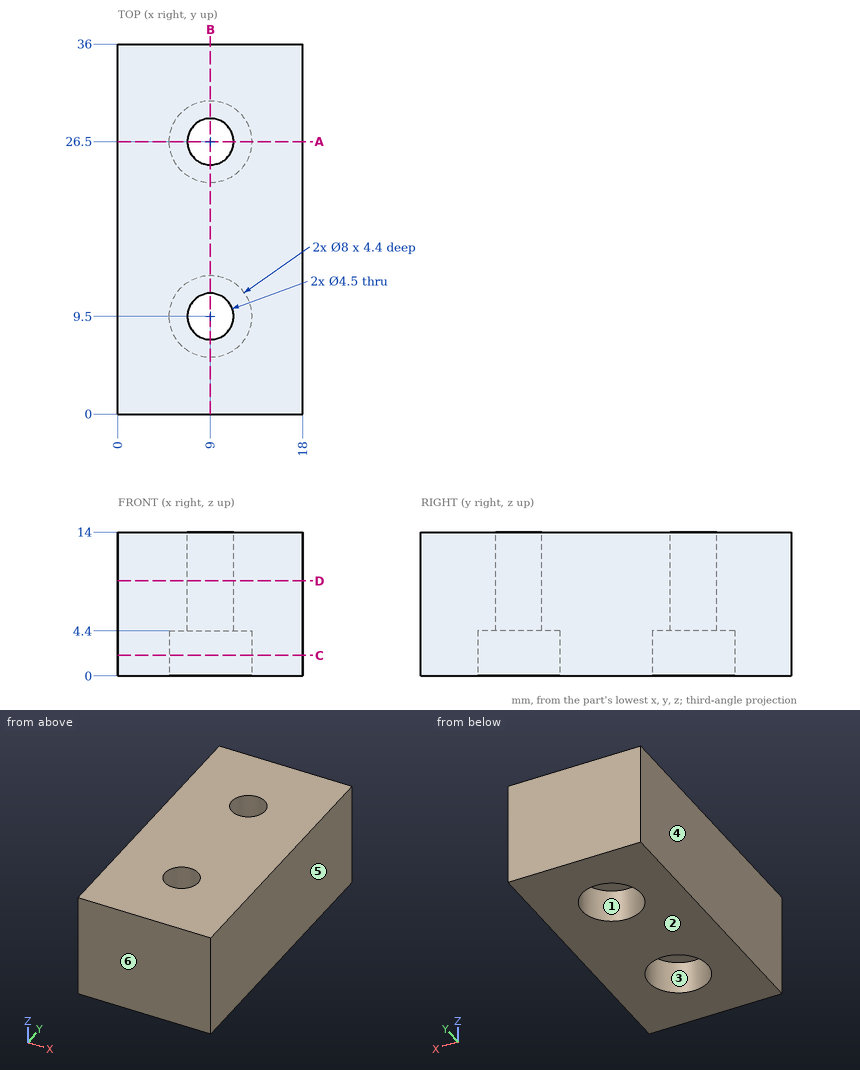
The figure shows three views and two pictorial views of one solid part (mm, origin at its lowest corner). Answer the questions. A direction names the side the tool comes from. Round coordinates to 2 decimals unless told otherwise and drop trailing zeros. Write each loop counter-clockwise with the first axis right and the second up, starting at its lowest first coordinate (ties: lowest second). Pieces come first, ordered by that corner, then holes. Notation, with made-up numbers: (-30, 0.5) -> (8, 0.5) arc R19 cw to (8, 25.5) -> close; hole circle Ø11 at (18.25, 37.5). An arc over 180 degrees is marked (long way). Answer as a JSON object with one key per item and string values. Group by question number.
Q1. Section A-A (y = 26.5) is taken. Write down the section's boundary in (x, z).
Q2. Which of the six approach directions +Z, -Z, +X, -X, +Y, -Y give full straight-line access (tool end or side, diameter ignored) to the marked faces 1 and 2?
Q3. This flat-tipped pin is pushed along its axis until it touches: pin 1 Ø7 at (x, y) = (9, 26.5) entering from -Z. Where does it stop, or does it pass through?
Q4. Section C-C (z = 2) is taken. Write down the section's boundary in (x, y).
Q5. Determine the mould class of the marked faces 3, 4, 5 and 6 for opening direction X: pulls with the +X half, pulls with the -X half, needs draft (parallel to the pull), parting line crosses it, or undercut.
Q6. Section B-B (x = 9) is taken. Write down the section's boundary in (y, z).
Q7. Section D-D (z = 9.25) is taken. Write down the section's boundary in (x, y), plus the area to 3 significant figures.
Q8. Straight lines are drawn through the part: line 1 along Y through (x, z) = (9, 2.05); line 2 along Y through (x, z) = (9, 9.5); line 3 along X through (y, z) = (29.5, 1.75). For each, find the intervals that lie inside material, in ascending order.
Check values:
{
 "1": {"outline": "(0, 0) -> (5, 0) -> (5, 4.4) -> (6.75, 4.4) -> (6.75, 14) -> (0, 14) -> close; (11.25, 4.4) -> (13, 4.4) -> (13, 0) -> (18, 0) -> (18, 14) -> (11.25, 14) -> close"},
 "2": {"face 1": "-Z", "face 2": "-Z, +X, -X, +Y, -Y"},
 "3": {"pin 1": "z = 4.4"},
 "4": {"outline": "(0, 0) -> (18, 0) -> (18, 36) -> (0, 36) -> close; hole circle Ø8 at (9, 9.5); hole circle Ø8 at (9, 26.5)"},
 "5": {"face 3": "undercut", "face 4": "pulls with the -X half", "face 5": "pulls with the +X half", "face 6": "needs draft"},
 "6": {"outline": "(0, 0) -> (5.5, 0) -> (5.5, 4.4) -> (7.25, 4.4) -> (7.25, 14) -> (0, 14) -> close; (11.75, 4.4) -> (13.5, 4.4) -> (13.5, 0) -> (22.5, 0) -> (22.5, 4.4) -> (24.25, 4.4) -> (24.25, 14) -> (11.75, 14) -> close; (28.75, 4.4) -> (30.5, 4.4) -> (30.5, 0) -> (36, 0) -> (36, 14) -> (28.75, 14) -> close"},
 "7": {"outline": "(0, 0) -> (18, 0) -> (18, 36) -> (0, 36) -> close; hole circle Ø4.5 at (9, 9.5); hole circle Ø4.5 at (9, 26.5)", "area": "616 mm^2"},
 "8": {"line 1": "0 to 5.5, 13.5 to 22.5, 30.5 to 36", "line 2": "0 to 7.25, 11.75 to 24.25, 28.75 to 36", "line 3": "0 to 6.35, 11.65 to 18"}
}
